Verification items for the finished model (mm, model axes). A direction names the side the tool comes from. Give positions to 0.01 mm unless a question says otherwise; leave off trailing zeros. Write each loop counter-clockwise with the first axis right and the second up, starting at its lowest first coordinate (ties: lowest second). Pieces come first, ordered by that corner, then holes. Notation, with made-up numbers: (11.25, -2.5) -> (65.25, -2.5) arc R14 ccw to (65.25, 17.5) -> close; hole circle Ø5 at (-9, 82.25). An arc over 180 degrees is marked (long way). Use one line per item in the form item = value. Start each with the question number.
(1) Release check for a two-part mould opening along X. For faces 1 (the face through (15, 1.3, -1.3)), 2 (the face through (-4, 0, -2)), 3 (the face through (-3.014, 1.293, -0.76)) record: pulls with the +X half, pulls with the -X half, needs draft (parallel to the pull), parting line crosses it, or undercut.
(2) Section check B-B, the plane x = 9.75. Record the cut outline in (y, z), plus the area to 3 significant figures.
(3) Scan lines: L1, parallel to X at y = 1.5, z = 1.5; L2, parallel to X at y = 1.25, z = 3.75; L3, parallel to Z at x = 0.75, y = 0.75. Record each from-to range of solid material in increasing order.
(4) Depth check by flat-ended pin: pin 1 Ø4 at (x, y) = (6, -2.5) entering from +Z; pin 2 Ø4 at (y, z) = (-3.5, -3.5) entering from -X; pin 3 Ø5 at (x, y) = (18.5, 2) entering from +Z. Enter the tip coordinate at first touch or a pass-through.
(5) Section check A-A, the plane x = 20. Record the cut outline in (y, z), plus the area to 3 significant figures.
(6) Set-up check for faces 4 (the face through (19, 0, -2)), 5 (the face through (-3, 0, -1.5)), 6 (the face through (-1.75, -0.59, 4.46)): record each of +Z, -Z, +X, -X, +Y, -Y from which the full face is reachable in a straight line by a thin tool's end or side.
Autodesk Inventor part; units mm, degrees
ref_plane "YZ Plane" through (0, 0, 0) normal (1, 0, 0) x (0, 1, 0)
ref_plane "XZ Plane" through (0, 0, 0) normal (0, 1, 0) x (-1, 0, 0)
ref_plane "XY Plane" through (0, 0, 0) normal (0, 0, 1) x (1, 0, 0)
sketch "Sketch_7" plane through (0, 0, 0) normal (0, 0, 1) x (1, 0, 0)
  line L0 (22, 0) -> (-1.134, 0)
  line L1 (-1.134, 0) -> (-2, 1.5)
  line L2 (-2, 1.5) -> (-4, 1.5)
  line L3 (-4, 1.5) -> (-4, 4.05)
  line L4 (-4, 4.05) -> (-3.55, 4.5)
  line L5 (-3.55, 4.5) -> (0, 4.5)
  line L6 (0, 4.5) -> (0, 3.25)
  arc A0 (0, 3.25) -> (0.7, 2.7) centre (0.5749, 3.2612) ccw
  line L7 (0.7, 2.7) -> (1, 3)
  line L8 (1, 3) -> (15, 3)
  line L9 (15, 3) -> (15, 1.5)
  line L10 (15, 1.5) -> (15.7, 1.5)
  line L11 (15.7, 1.5) -> (16.2, 2)
  line L12 (16.2, 2) -> (21.5705, 2)
  line L13 (21.5705, 2) -> (22, 1.5705)
  line L14 (22, 1.5705) -> (22, 0)
  line L15 (22, 0) -> (-1.134, 0)
revolve "Revolution1" add sketch "Sketch_7" angle 360 about axis through (22, 0, 0) along (1, 0, 0)
thread "Thread1"
sketch "Sketch_4" plane through (-4, 0, 0) normal (1, 0, 0) x (0, 0, -1)
  line L0 (-1.5, -0.866) -> (0, -1.7321)
  line L1 (0, -1.7321) -> (1.5, -0.866)
  line L2 (1.5, -0.866) -> (1.5, 0.866)
  line L3 (1.5, 0.866) -> (0, 1.7321)
  line L4 (0, 1.7321) -> (-1.5, 0.866)
  line L5 (-1.5, 0.866) -> (-1.5, -0.866)
extrude "Extrusion1" cut sketch "Sketch_4" along normal blind 2
properties part number "MSB6-15" material "鋼、炭素鋼"
Completed:
q1.face_1 = undercut
q1.face_2 = pulls with the -X half
q1.face_3 = needs draft
q2.outline = circle Ø6 at (0, 0)
q2.area = 28.3 mm²
q3.L1 = -4 to 15
q3.L2 = -4 to 0
q3.L3 = -2.65 to 2.65
q4.pin_1 = 2.96
q4.pin_2 = -4
q4.pin_3 = 2
q5.outline = circle Ø4 at (0, 0)
q5.area = 12.6 mm²
q6.face_4 = +X
q6.face_5 = -X
q6.face_6 = +X, -X
